For this review, use the dimensioned drawing (mm, ordinates from the lowest corner) and the shaded views. A direction names the side the tool comes from. Round coordinates to 2 decimals unless told otherwise and drop trailing zeros. Loops run counter-clockwise (first coordinate to the right, second up) from the corner with the lowest first, then second, coordinate; pieces in that order, holes last. Notation, with made-up numbers: (-31, 9.5) -> (-13, 9.5) arc R30 cw to (-13, 32.5) -> close; hole circle Ø9 at (55.25, 57.25). An arc over 180 degrees is marked (long way). Use one line per item in the form item = value. Start each with the question number.
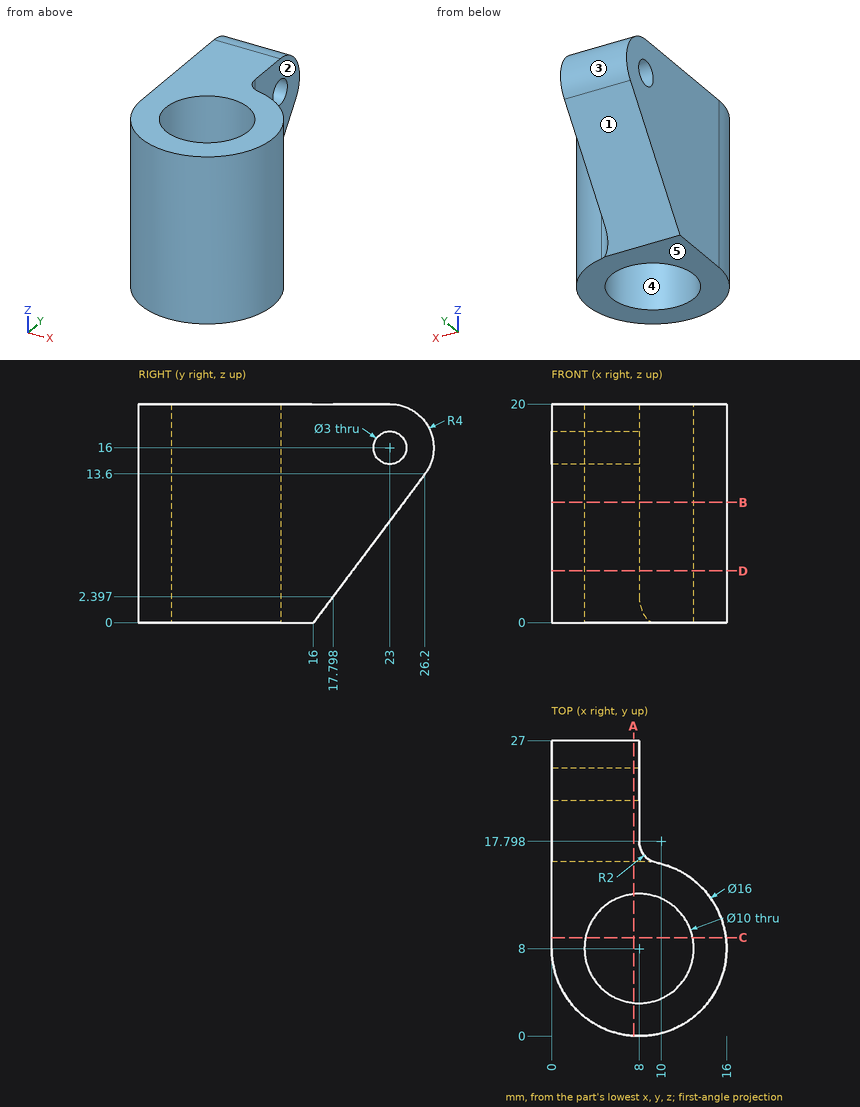
Item 1: Take a section at C-C on y = 9. Give the boundary of the cut face in (x, z).
Item 2: Take a section at B-B on z = 11. Give the boundary of the cut face in (x, y).
Item 3: For P1, Ø2, axis at x = 5, z = 3.5, coming from the -Y side; P2, Ø1.5, axis at x = 11, z = 8.5, coming from the +Y side; P3, Ø8, axis at y = 5.5, z = 14.5, coming from the -X side; P4, Ø3, axis at y = 10.5, z = 5.5, coming from the +X side, all flat-tipped, find the tip position at first contact; note any pin that passes through.
Item 4: Draft analysis for pull direction Y (two halves, no side actions). For the marked faces 3, 4 and 5, state which applies: +Y half, -Y half, draft (parallel to the pull), parting line (faces both ways), or undercut.
Item 5: Take a section at D-D on z = 4.75. Give the boundary of the cut face in (x, y), plus the area to 3 significant figures.
Item 6: Machinability: for the marked faces 1 and 2, which of the approach directions +Z, -Z, +X, -X, +Y, -Y give a long, thin tool a straight path to every point of the face, cutting with its end or side? Answer none if there is none.
Item 7: Wall thickness on line 1 (X direction, y = 20.75, z = 18.5); line 2 (Y direction, x = 3.5, z = 16) (1 decimal); line 3 (X direction, y = 12, z = 3.5): over which ranges is each line inside the solid? List them lowest first.
Item 8: Take a section at A-A on x = 7.5. Give the boundary of the cut face in (y, z) (1 decimal), plus the area to 3 significant figures.
Results:
q1.outline = (0, 0) -> (3.1, 0) -> (3.1, 20) -> (0, 20) -> close; (12.9, 0) -> (15.94, 0) -> (15.94, 20) -> (12.9, 20) -> close
q2.outline = (0, 8) arc R8 ccw (long way) to (9.6, 15.84) arc R2 cw to (8, 17.8) -> (8, 24.25) -> (0, 24.25) -> close; hole circle Ø10 at (8, 8)
q3.P1 = 0.25
q3.P2 = 15.68
q3.P3 = 0
q3.P4 = 15.94
q4.face_3 = +Y half
q4.face_4 = undercut
q4.face_5 = draft
q5.outline = (0, 8) arc R8 ccw (long way) to (9.6, 15.84) arc R2 cw to (8, 17.8) -> (8, 19.56) -> (0, 19.56) -> close; hole circle Ø10 at (8, 8)
q5.area = 165 mm2
q6.face_1 = -Z, +X, -X, +Y
q6.face_2 = +Z, -Z, +X, +Y
q7.line_1 = 0 to 8
q7.line_2 = 1.4 to 5.8, 10.2 to 21.5, 24.5 to 27
q7.line_3 = 0 to 5, 11 to 14.93
q8.outline = (0, 0) -> (3, 0) -> (3, 20) -> (0, 20) -> close; (13, 0) -> (16, 0) -> (26.2, 13.6) arc R4 ccw to (23, 20) -> (13, 20) -> close; hole circle Ø3 at (23, 16)
q8.area = 249 mm2
